Geometry check sheet. Reference: the model listing, model coordinates, mm. Face numbers are marked on the shaded views. Coordinates: 2 decimals unless noted, no trailing zeros. Order: outer loops, then holes, each group sorted by start corner. A loop starts at its lowest first (then second) coordinate and runs counter-clockwise, first axis right, second up. Notation, with made-up numbers: (30, 34.5) -> (68, 34.5) arc R23 ccw to (68, 47.5) -> close; hole circle Ø10 at (15, -14). An arc over 180 degrees is marked (long way). Answer in a Markdown table with one row per item. Add a question column.
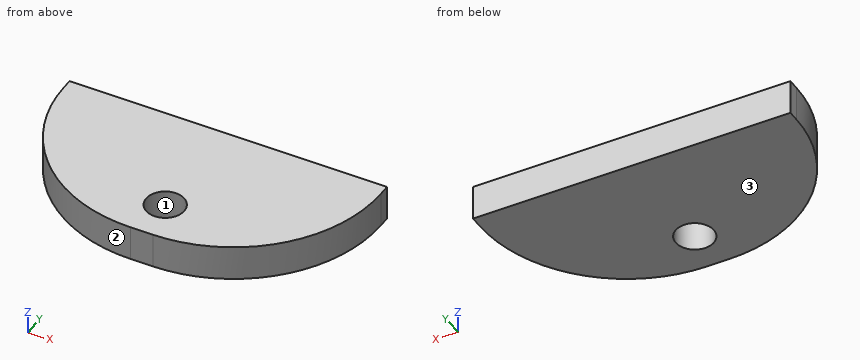
```python
from build123d import *

# Parameters (mm, degrees)
BOX002_W        = 28
BOX002_H        = 14
BOX002_DEPTH    = 3.1
SKETCH017_R     = 1.68
POCKET009_DEPTH = 5
FILLET003_R     = 13


with BuildPart() as part:
    # Box002 → Box002 (new body)
    with BuildSketch(Plane(origin=(12, -13, 0), x_dir=(1, 0, 0), z_dir=(0, 0, 1))):
        with Locations((14, 7)):
            Rectangle(BOX002_W, BOX002_H)
    extrude(amount=BOX002_DEPTH)

    # Sketch017 → Pocket009 (cut)
    with BuildSketch(Plane(origin=(12, -13, 0), x_dir=(1, 0, 0), z_dir=(0, 0, -1))):
        with Locations((14, -3.8)):
            Circle(SKETCH017_R)
    extrude(amount=-POCKET009_DEPTH, mode=Mode.SUBTRACT)

    # Fillet003
    fillet003_edges = [part.edges().sort_by_distance(p)[0] for p in [
        (40, -13, 1.55),
        (12, -13, 1.55),
    ]]
    fillet(fillet003_edges, radius=FILLET003_R)


solid = part.part
```
(1) Cross-section at A-A (z = 2.05). Enter the section's corners in (x, y).
(2) Scan lines: line 1 along Y through (x, z) = (26, 1.95); line 2 along X through (y, z) = (-10, 1.9); line 3 along X through (y, z) = (-0.25, 2.3). Record each from-to range of solid material in increasing order.
(3) Cross-section at D-D (y = -5.75). Enter the section's corners in (x, z), plus the area to 3 significant figures.
(4) Mould release check, pull along Y, two halves, no side actions. Record for the marked faces 1, 2 and 3: +Y half, -Y half, draft (parallel to the pull), parting line (faces both ways), or undercut.
(5) Go/stop test with a flat-tipped pin: P1, Ø1, axis at y = -4, z = 2, coming from the -X side. Record where the tip stops, or that it passes through.
(6) Cross-section at B-B (x = 26). Enter the section's corners in (y, z).
(7) Cross-section at C-C (y = -10.5). Enter the section's corners in (x, z).
Checks:
| question | item | result |
|---|---|---|
| 1 | outline | (12, 0) arc R13 ccw to (25, -13) -> (27, -13) arc R13 ccw to (40, 0) -> (40, 1) -> (12, 1) -> close; hole circle Ø3.36 at (26, -9.2) |
| 2 | line 1 | -13 to -10.88, -7.52 to 1 |
| 2 | line 2 | 16.69 to 24.52, 27.48 to 35.31 |
| 2 | line 3 | 12 to 40 |
| 3 | outline | (13.34, 0) -> (38.66, 0) -> (38.66, 3.1) -> (13.34, 3.1) -> close |
| 3 | area | 78.5 mm² |
| 4 | face 1 | undercut |
| 4 | face 2 | -Y half |
| 4 | face 3 | draft |
| 5 | P1 | x = 12.48 |
| 6 | outline | (-13, 0) -> (-10.88, 0) -> (-10.88, 3.1) -> (-13, 3.1) -> close; (-7.52, 0) -> (1, 0) -> (1, 3.1) -> (-7.52, 3.1) -> close |
| 7 | outline | (17.34, 0) -> (24.94, 0) -> (24.94, 3.1) -> (17.34, 3.1) -> close; (27.06, 0) -> (34.66, 0) -> (34.66, 3.1) -> (27.06, 3.1) -> close |
